Geometry check sheet. Reference: the model listing, model coordinates, mm. Coordinates: 2 decimals unless noted, no trailing zeros. Order: outer loops, then holes, each group sorted by start corner. A loop starts at its lowest first (then second) coordinate and runs counter-clockwise, first axis right, second up.
```python
from build123d import *

# Parameters (mm, degrees)
SZKIC1_R                                    = 150
DODANIE_WYCI_GNI_CIE1_DEPTH                 = 6
OTWORY_USTALAJ_CE_8_0MM1_D                  = 8
OTWORY_USTALAJ_CE_8_0MM1_CSINK_D            = 8.05
OTWORY_USTALAJ_CE_8_0MM1_CSINK_ANGLE        = 90
POG_BIENIE_STO_KOWE_POD_M8_WKR_T_DO_2_COUNT = 2
POG_BIENIE_STO_KOWE_POD_M8_WKR_T_DO_2_PITCH = 190.91883092
POG_BIENIE_STO_KOWE_POD_M8_WKR_T_DO_3_COUNT = 2
POG_BIENIE_STO_KOWE_POD_M8_WKR_T_DO_3_PITCH = 270
POG_BIENIE_STO_KOWE_POD_M8_WKR_T_DO_4_COUNT = 2
POG_BIENIE_STO_KOWE_POD_M8_WKR_T_DO_4_PITCH = 190.91883092


with BuildPart() as part:
    # Szkic1 → Dodanie-wyciągnięcie1 (new body)
    with BuildSketch(Plane.XY):
        Circle(SZKIC1_R)
    extrude(amount=DODANIE_WYCI_GNI_CIE1_DEPTH)

    # Otwory ustalające Ø8.0mm1 (through all)
    with Locations(Plane.XY.offset(6)):
        with Locations((0, 60), (0, -60)):
            CounterSinkHole(OTWORY_USTALAJ_CE_8_0MM1_D / 2, OTWORY_USTALAJ_CE_8_0MM1_CSINK_D / 2, counter_sink_angle=OTWORY_USTALAJ_CE_8_0MM1_CSINK_ANGLE)

    # Szkic6 → Otwory ustalające Ø12.0mm1 (revolve, cut)
    with BuildSketch(Plane(origin=(0, 0, 6), x_dir=(0, -1, 0), z_dir=(1, 0, 0))):
        Polygon((0, 0), (0, 6), (6, 6), (6, 0.025), (6.025, 0), align=None)
    revolve(axis=Axis((0, 0, 12.35), (0, 0, -1)), mode=Mode.SUBTRACT)

    # Szkic10 → Pogłębienie stożkowe pod M8 wkręt do części metalowych z łbem soczewkowym1 (revolve, cut)
    with BuildSketch(Plane(origin=(0, 135, 6), x_dir=(0, -1, 0), z_dir=(1, 0, 0))):
        Polygon((0, 0), (0, 6), (4.5, 6), (4.5, 4.15), (8.65, 0), align=None)
    pog_bienie_sto_kowe_pod_m8_wkr_t_do_cz_c = revolve(axis=Axis((0, 135, 12.35), (0, 0, -1)), mode=Mode.SUBTRACT)

    # Pog_bienie sto_kowe pod M8 wkr_t do  2: Pogłębienie stożkowe pod M8 wkręt do części metalowych z łbem soczewkowym1 ×2
    with Locations(*[Vector(0.7071067811865674, -0.7071067811865276, 0) * (i * POG_BIENIE_STO_KOWE_POD_M8_WKR_T_DO_2_PITCH) for i in range(1, POG_BIENIE_STO_KOWE_POD_M8_WKR_T_DO_2_COUNT)]):
        add(pog_bienie_sto_kowe_pod_m8_wkr_t_do_cz_c, mode=Mode.SUBTRACT)

    # Pog_bienie sto_kowe pod M8 wkr_t do  3: Pogłębienie stożkowe pod M8 wkręt do części metalowych z łbem soczewkowym1 ×2
    with Locations(*[(0, -i * POG_BIENIE_STO_KOWE_POD_M8_WKR_T_DO_3_PITCH, 0) for i in range(1, POG_BIENIE_STO_KOWE_POD_M8_WKR_T_DO_3_COUNT)]):
        add(pog_bienie_sto_kowe_pod_m8_wkr_t_do_cz_c, mode=Mode.SUBTRACT)

    # Pog_bienie sto_kowe pod M8 wkr_t do  4: Pogłębienie stożkowe pod M8 wkręt do części metalowych z łbem soczewkowym1 ×2
    with Locations(*[Vector(-0.7071067811865277, -0.7071067811865674, 0) * (i * POG_BIENIE_STO_KOWE_POD_M8_WKR_T_DO_4_PITCH) for i in range(1, POG_BIENIE_STO_KOWE_POD_M8_WKR_T_DO_4_COUNT)]):
        add(pog_bienie_sto_kowe_pod_m8_wkr_t_do_cz_c, mode=Mode.SUBTRACT)


solid = part.part
```
Item 1: Sectioned sample at C-C (x = -135). Record the cut outline in (y, z), and give its area (3 significant figures).
Item 2: Sectioned sample at B-B (z = 5). Record the cut outline in (x, y), and give its area (3 significant figures).
Item 3: Depth check by flat-ended pin: P1, Ø11.5, axis at x = 0, y = -135, coming from the +Z side; P2, Ø1.5, axis at y = 26.5, z = 2, coming from the -X side; P3, Ø1.5, axis at y = 73.5, z = 1.5, coming from the +X side. Enter the tip coordinate at first touch or a pass-through.
Item 4: Sectioned sample at A-A (y = 0). Record the cut outline in (x, z) (3 decimals), and give its area (3 significant figures).
Item 5: Release check for a two-part mould opening along Y. For faces 1 (the face through (0, 6, 3)), 2 (the face through (136.82, -4.4, 2.11)), 3 (the face through (-2, -31, 0)), 4 (the face through (-19.527, 148.724, 2.958)) record: pulls with the +Y half, pulls with the -Y half, needs draft (parallel to the pull), parting line crosses it, or undercut.
Item 6: Thickness scan on line 1 along Y through (x, z) = (0, 1.5); line 2 along Y through (x, z) = (0, 3.1); line 3 along X through (y, z) = (60, 3.05). Record the ranges inside material, lowest first.
Geometry check:
1. outline: (-65.38, 0) - (-4.5, 0) - (-4.5, 1.85) - (-8.65, 6) - (-65.38, 6) - close; (4.5, 0) - (65.38, 0) - (65.38, 6) - (8.65, 6) - (4.5, 1.85) - close
1. area: 713 mm2
2. outline: circle Ø300 at (0, 0); hole circle Ø15.3 at (-135, 0); hole circle Ø15.3 at (0, -135); hole circle Ø15.3 at (0, 135); hole circle Ø12 at (0, 0); hole circle Ø8 at (0, -60); hole circle Ø8 at (0, 60); hole circle Ø15.3 at (135, 0)
2. area: 69,700 mm2
3. P1: stops at z = 3.1
3. P2: stops at x = -147.77
3. P3: stops at x = 131.18
4. outline: (-150, 0) - (-139.5, 0) - (-139.5, 1.85) - (-143.65, 6) - (-150, 6) - close; (-130.5, 0) - (-6, 0) - (-6, 5.975) - (-6.025, 6) - (-126.35, 6) - (-130.5, 1.85) - close; (6, 0) - (130.5, 0) - (130.5, 1.85) - (126.35, 6) - (6.025, 6) - (6, 5.975) - close; (139.5, 0) - (150, 0) - (150, 6) - (143.65, 6) - (139.5, 1.85) - close
4. area: 1,590 mm2
5. face 1: undercut
5. face 2: undercut
5. face 3: needs draft
5. face 4: parting line crosses it
6. line 1: y = -150 to -139.5, -130.5 to -64, -56 to -6, 6 to 56, 64 to 130.5, 139.5 to 150
6. line 2: y = -150 to -140.75, -129.25 to -64, -56 to -6, 6 to 56, 64 to 129.25, 140.75 to 150
6. line 3: x = -137.48 to -4, 4 to 137.48
